```python
from build123d import *

# Parameters (mm, degrees)
EXTRUDE_2_DEPTH = 4


with BuildPart() as part:
    # Эскиз3 → Бобышка-Вытянуть2 (new body)
    with BuildSketch(Plane(origin=(0, 0, 0), x_dir=(1, 0, 0), z_dir=(0, 1, 0))):
        Polygon((110, -32), (110, 23), (95, 23), (95, 27), (85, 27), (85, 23), (75, 23), (75, 27), (65, 27), (65, 23), (55, 23), (55, 27), (45, 27), (45, 23), (35, 23), (35, 27), (25, 27), (25, 23), (15, 23), (15, 27), (5, 27), (5, 23), (-5, 23), (-5, 27), (-15, 27), (-15, 23), (-25, 23), (-25, 27), (-35, 27), (-35, 23), (-45, 23), (-45, 27), (-55, 27), (-55, 23), (-65, 23), (-65, 27), (-75, 27), (-75, 23), (-85, 23), (-85, 27), (-95, 27), (-95, 23), (-110, 23), (-110, -32), (-95, -32), (-95, -36), (-85, -36), (-85, -32), (-75, -32), (-75, -36), (-65, -36), (-65, -32), (-55, -32), (-55, -36), (-45, -36), (-45, -32), (-35, -32), (-35, -36), (-25, -36), (-25, -32), (-15, -32), (-15, -36), (-5, -36), (-5, -32), (5, -32), (5, -36), (15, -36), (15, -32), (25, -32), (25, -36), (35, -36), (35, -32), (45, -32), (45, -36), (55, -36), (55, -32), (65, -32), (65, -36), (75, -36), (75, -32), (85, -32), (85, -36), (95, -36), (95, -32), align=None)
    extrude(amount=EXTRUDE_2_DEPTH)


solid = part.part
```
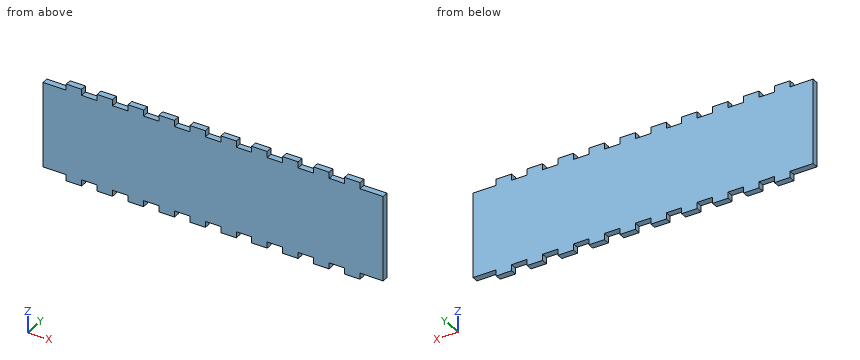
CAD build for the part. Positions are in the model's coordinates, mm. Give positions to 0.01 mm unless a question says otherwise; leave off trailing zeros. Write each loop counter-clockwise with the first axis right and the second up, starting at its lowest first coordinate (ties: lowest second). Pieces come first, ordered by that corner, then holes. Notation, with made-up numbers: (62.5, 79) -> (71.5, 79) arc R11 ccw to (71.5, 99) -> close; hole circle Ø2 at (82, -29.75). An arc over 180 degrees is marked (long way). Write each question's results on one line, items separated by ' | '.
1. Drop flat-ended pins along their axis: P1, Ø1.2, axis at x = 39, y = 1, coming from the -Z side; P2, Ø1.2, axis at y = 1.5, z = -24.5, coming from the -X side; P3, Ø8, axis at x = -59, z = -13, coming from the -Y side; P4, Ø1.2, axis at y = 2, z = -25.5, coming from the +X side. Give the stop position or say it passes through.
Geometry check:
P1: z = -23 | P2: x = -95 | P3: y = 0 | P4: x = 95
2. Wall check: probe 1 along Z at (x, y) = (-97, 2.1). Give the ranges that are in metal, low to high. Write a range as [from, to].
Geometry check:
probe 1: [-23, 32]
3. Cut at A-A, the plane x = 63. Write the cut outline in (y, z).
Geometry check:
outline: (0, -23) -> (4, -23) -> (4, 32) -> (0, 32) -> close
